from build123d import *

# Parameters (mm, degrees)
F1_DEPTH = 12.7
F2_SIZE2 = 38.1
F2_SIZE  = 38.1
F4_D     = 6.35
F6_D     = 3.96875


with BuildPart() as f1:
    # F0 (on Front) → F1 (new body)
    with BuildSketch(Plane.XZ):
        with BuildLine():
            Line((711.2, 78.1812), (711.2, 0))
            Line((711.2, 0), (1473.2, 0))
            Line((1473.2, 0), (1473.2, 562.7624))
            Line((1473.2, 562.7624), (711.2, 562.7624))
            Line((711.2, 562.7624), (711.2, 484.5812))
            ThreePointArc((711.2, 484.5812), (688.881537, 430.699663), (635, 408.3812))
            Line((635, 408.3812), (0, 408.3812))
            Line((0, 408.3812), (0, 154.3812))
            Line((0, 154.3812), (635, 154.3812))
            ThreePointArc((635, 154.3812), (688.881537, 132.062737), (711.2, 78.1812))
        make_face()
    extrude(amount=F1_DEPTH)

    # F2
    f2_edges = [f1.edges().sort_by_distance(p)[0] for p in [
        (711.2, -6.35, 562.7624),
        (711.2, -6.35, 0),
        (1473.2, -6.35, 0),
        (1473.2, -6.35, 562.7624),
        (0, -6.35, 154.3812),
        (0, -6.35, 408.3812),
    ]]
    chamfer(f2_edges, length=F2_SIZE, length2=F2_SIZE2)

    # F4 (through all)
    with Locations(Plane.XZ.offset(12.7)):
        with Locations((1092.2, 215.9), (1092.2, 346.8624), (1282.7, 346.8624), (1282.7, 215.9)):
            Hole(F4_D / 2)

    # F6 (through all)
    with Locations(Plane.XZ.offset(12.7)):
        with Locations((749.293897, 545.3126), (749.293897, 502.4374), (774.693897, 502.4374), (774.693897, 545.3126), (749.293897, 60.325), (774.693897, 17.4498), (749.293897, 17.4498), (774.693897, 60.325), (1409.706103, 502.4374), (1435.106103, 502.4374), (1435.106103, 545.3126), (1409.706103, 545.3126), (1409.706103, 17.4498), (1435.106103, 17.4498), (1435.106103, 60.325), (1409.706103, 60.325)):
            Hole(F6_D / 2)


solid = f1.part
Geometry check sheet. Reference: the model listing, model coordinates, mm. Round coordinates to 2 decimals unless told otherwise and drop trailing zeros. Write each loop counter-clockwise with the first axis right and the second up, starting at its lowest first coordinate (ties: lowest second). Pieces come first, ordered by that corner, then holes. Notation, with made-up numbers: (16, 50) -> (50, 50) arc R9 ccw to (50, 55) -> close; hole circle Ø2 at (51, 62.5). An arc over 180 degrees is marked (long way). One line per item, written item: value. Start each with the question number.
(1) Scan lines: line 1 (Z direction, x = 1282.7, y = -7.25) (3 decimals); line 2 (X direction, y = -1.25, z = 346); line 3 (Z direction, x = 350, y = -11). Record each from-to range of solid material in increasing order. Write a range as [from, to].
(2) Cross-section at B-B, the plane y = -7.25. Give the number of separate pieces and of enclosed holes in the cut face, and give its area (3 significant figures).
(3) Cross-section at A-A, the plane x = 226. Record the cut outline in (y, z), and give its area (3 significant figures).
(4) Go/stop test with flat-tipped pins: pin 1 Ø2 at (x, y) = (621.5, -9.5) entering from -Z; pin 2 Ø1.5 at (y, z) = (-7.5, 156) entering from -X. Record where each tip stops, or that it passes through.
(5) Cross-section at C-C, the plane z = 459. Record the cut outline in (x, y).
Answer:
1. line 1: [0, 212.725], [219.075, 343.687], [350.037, 562.762]
1. line 2: [0, 1089.14], [1095.26, 1279.64], [1285.76, 1473.2]
1. line 3: [154.38, 408.38]
2. separate pieces: 1
2. enclosed holes: 20
2. area: 607,000 mm²
3. outline: (-12.7, 154.38) -> (0, 154.38) -> (0, 408.38) -> (-12.7, 408.38) -> close
3. area: 3,230 mm²
4. pin 1: z = 154.38
4. pin 2: x = 35.73
5. outline: (706.78, -12.7) -> (1473.2, -12.7) -> (1473.2, 0) -> (706.78, 0) -> close
